The listing builds one solid part. Answer for the finished solid, in the listing's coordinates (mm). A direction names the side the tool comes from. Round coordinates to 2 decimals unless told otherwise and drop trailing zeros. Write each loop counter-clockwise with the first axis right and the second up, starting at its lowest first coordinate (ties: lowest second). Pieces come first, ordered by that corner, then holes.
Item 1: For a pull along X with two mould halves and no side action, classify faces 1 (the face through (-211.96, 338.15, -1.46)), 2 (the face through (-215.666, 348.43, 0.132)), 3 (the face through (-216, 345, -27)) as +X half, -X half, draft (parallel to the pull), parting line (faces both ways), or undercut.
Item 2: Find section A-A on z = -20.5. Give the vertices of the cut face in (x, y).
Item 3: A tool of negligible diameter and unlimited length cuts with its end or side. For faces 4 (the face through (-220.521, 341.106, -15.139)), 5 (the face through (-225.44, 350.18, -3.01)), 6 (the face through (-212.991, 339.434, 15.466)), from which of +Z, -Z, +X, -X, +Y, -Y can it reach the whole face along a straight path? Write none if from no direction.
Item 4: Find the intervals of material crossed by probe 1 along Z at (x, y) = (-222, 351.5); probe 2 along Z at (x, y) = (-224.25, 349.25); probe 3 along X at (y, z) = (341, 15.5), in increasing order.
Item 5: Each of these flat-tipped pins is pushed along its axis until it touches: pin 1 (12 mm diameter, centred on y = 341.5, z = -12.5, fed in from +X); pin 2 (5 mm diameter, centred on y = 338, z = -13, fed in from +X); pin 3 (10 mm diameter, centred on x = -211, y = 354, fed in from +Z); pin 4 (6 mm diameter, centred on y = 345, z = -10.5, fed in from +X). Where does it stop, or does it pass through?
```python
from build123d import *

# Parameters (mm, degrees)
PUENTE_PROFILE_R           = 6
BOSS_TORNILLO_PROFILE_R    = 7
TALADRO_TORNILLO_PROFILE_R = 3


with BuildPart() as part:
    # Puente: sweep along a curve in space
    with BuildLine() as puente_path:
        Line((-215.759160386, 344.756610234, -27), (-215.759160386, 344.756610234, 27))
    # Puente profile (on start of the path) → Puente (sweep)
    with BuildSketch(Plane(origin=(-215.759160386, 344.756610234, -27), x_dir=(1, 0, 0), z_dir=(0, 0, 1))):
        Circle(PUENTE_PROFILE_R)
    sweep(path=puente_path.line)

    # Boss_tornillo: sweep along a curve in space
    with BuildLine() as boss_tornillo_path:
        Line((-210.15458046, 340.562723747, 0), (-224.566357411, 351.347003284, 0))
    # Boss_tornillo profile (on start of the path) → Boss_tornillo (sweep)
    with BuildSketch(Plane(origin=(-210.15458046, 340.562723747, 0), x_dir=(-0.5991266409502979, -0.8006542750173841, 0), z_dir=(-0.8006542750173841, 0.5991266409502979, 0))):
        Circle(BOSS_TORNILLO_PROFILE_R)
    sweep(path=boss_tornillo_path.line)

    # Taladro_tornillo: sweep along a curve in space
    with BuildLine() as taladro_tornillo_path:
        Line((-209.353926185, 339.963597106, 0), (-225.367011686, 351.946129925, 0))
    # Taladro_tornillo profile (on start of the path) → Taladro_tornillo (sweep, cut)
    with BuildSketch(Plane(origin=(-209.353926185, 339.963597106, 0), x_dir=(-0.5991266409502969, -0.8006542750173848, 0), z_dir=(-0.8006542750173848, 0.5991266409502969, 0))):
        Circle(TALADRO_TORNILLO_PROFILE_R)
    sweep(path=taladro_tornillo_path.line, mode=Mode.SUBTRACT)


solid = part.part
```
Check values:
1. face 1: +X half
1. face 2: undercut
1. face 3: draft
2. outline: circle Ø12 at (-215.76, 344.76)
3. face 4: -Z
3. face 5: +Z, -Z, -X, +Y
3. face 6: +Z
4. probe 1: z = -6.8 to -2.5, 2.5 to 6.8
4. probe 2: z = -6.84 to -2.6, 2.6 to 6.84
4. probe 3: x = -220.44 to -211.08
5. pin 1: stops at x = -208.72
5. pin 2: stops at x = -211.53
5. pin 3: stops at z = 27
5. pin 4: stops at x = -209.76
